Design review of the part built by this model. Coordinates are the model's own, in mm. Face numbers are marked on the shaded views. Round coordinates to 2 decimals unless told otherwise and drop trailing zeros. Loops run counter-clockwise (first coordinate to the right, second up) from the corner with the lowest first, then second, coordinate; pieces in that order, holes last. Notation, with made-up numbers: (60, 23) -> (84, 23) arc R19 cw to (84, 39) -> close; hole circle Ø11 at (32.25, 22). An arc over 180 degrees is marked (long way). Use a Markdown table: item, result. Add a question column.
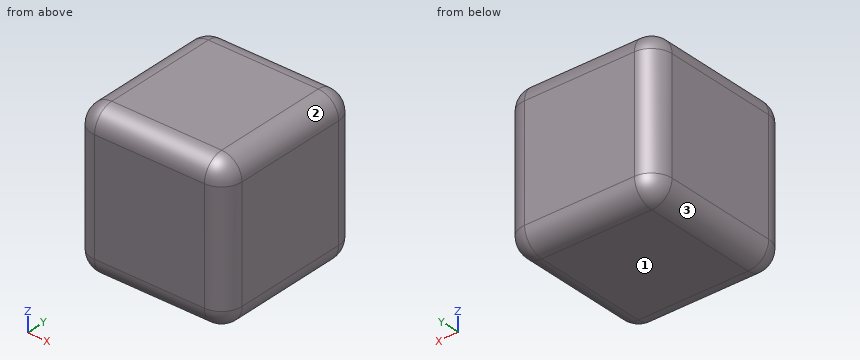
from build123d import *

# Parameters (mm, degrees)
F0_W     = 37.4110154808
F0_H     = 38.7368313968
F1_DEPTH = 38.1
F2_R     = 5.08
F3_R     = 5.08
F4_R     = 5.08
F5_R     = 5.08
F6_R     = 5.08
F7_R     = 5.08


# Not quite as in the source:
# - the program builds the solid bodies; features that only make, move or delete a surface that nothing else refers to are left out


with BuildPart() as f1:
    # F0 (on Top) → F1 (new body)
    with BuildSketch(Plane.XY):
        Rectangle(F0_W, F0_H)
    extrude(amount=F1_DEPTH)

    # F2
    f2_edges = [f1.edges().sort_by_distance(p)[0] for p in [
        (18.705508, -19.368416, 19.05),
    ]]
    fillet(f2_edges, radius=F2_R)

    # F3
    f3_edges = [f1.edges().sort_by_distance(p)[0] for p in [
        (-18.705508, -19.368416, 19.05),
    ]]
    fillet(f3_edges, radius=F3_R)

    # F4
    f4_edges = [f1.edges().sort_by_distance(p)[0] for p in [
        (-18.705508, 19.368416, 19.05),
    ]]
    fillet(f4_edges, radius=F4_R)

    # F5
    f5_edges = [f1.edges().sort_by_distance(p)[0] for p in [
        (18.705508, 19.368416, 19.05),
    ]]
    fillet(f5_edges, radius=F5_R)

    # F6
    f6_edges = [f1.edges().sort_by_distance(p)[0] for p in [
        (0, 19.368416, 38.1),
    ]]
    fillet(f6_edges, radius=F6_R)

    # F7
    f7_edges = [f1.edges().sort_by_distance(p)[0] for p in [
        (0, -19.368416, 0),
    ]]
    fillet(f7_edges, radius=F7_R)


solid = f1.part
1. Consider section B-B on y = -7.5. State the section outline as (x, z) points, plus the area to 3 significant figures.
2. Mouldability with a two-part tool opening along X and no side actions: class the marked faces 1, 2 and 3 as +X half, -X half, draft (parallel to the pull), parting line (faces both ways), or undercut.
3. To check wall thickness, follow probe 1 along X at (y, z) = (-4, 2.5); probe 2 along Z at (x, y) = (14, -14); probe 3 along Y at (x, z) = (-15, 18). State the ranges of each line that lie inside material, in increasing order. Write a range as from..to.
4. Consider section A-A on z = 10.5. State the section outline as (x, y) points, plus the area to 3 significant figures.
Verdict:
| question | item | result |
|---|---|---|
| 1 | outline | (-18.71, 5.08) arc R5.08 ccw to (-13.63, 0) -> (13.63, 0) arc R5.08 ccw to (18.71, 5.08) -> (18.71, 33.02) arc R5.08 ccw to (13.63, 38.1) -> (-13.63, 38.1) arc R5.08 ccw to (-18.71, 33.02) -> close |
| 1 | area | 1,400 mm² |
| 2 | face 1 | draft |
| 2 | face 2 | +X half |
| 2 | face 3 | -X half |
| 3 | probe 1 | x = -18..18 |
| 3 | probe 2 | z = 0.01..38.09 |
| 3 | probe 3 | y = -19.18..19.18 |
| 4 | outline | (-18.71, -14.29) arc R5.08 ccw to (-13.63, -19.37) -> (13.63, -19.37) arc R5.08 ccw to (18.71, -14.29) -> (18.71, 14.29) arc R5.08 ccw to (13.63, 19.37) -> (-13.63, 19.37) arc R5.08 ccw to (-18.71, 14.29) -> close |
| 4 | area | 1,430 mm² |
